Read the model definition and answer for the solid it produces. Units are mm, in the model's axes. Round coordinates to 2 decimals unless told otherwise and drop trailing zeros. Loops run counter-clockwise (first coordinate to the right, second up) from the corner with the lowest first, then second, coordinate; pieces in that order, holes last. Notation, with made-up numbers: (61.5, 60.5) - (115.5, 60.5) arc R21 ccw to (115.5, 78.5) - close; hole circle Ø2 at (25, -34). An arc over 180 degrees is marked (long way). Answer as CSV lines item,"result".
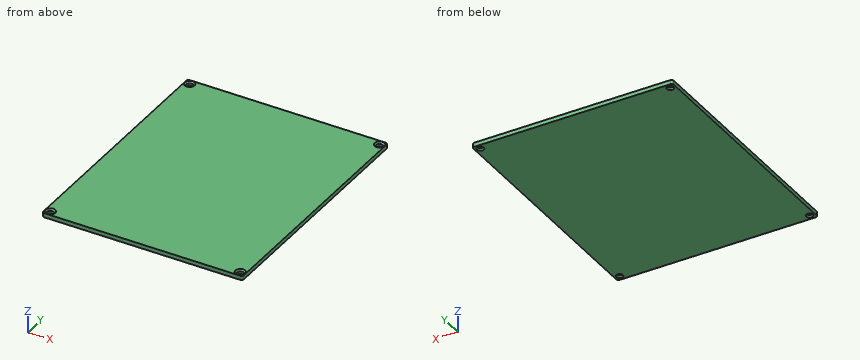
```python
from build123d import *

# Parameters (mm, degrees)
SKIZZE1_W                       = 96
SKIZZE1_H                       = 118
SKIZZE1_R                       = 1.6
AUFSATZ_LINEAR_AUSTRAGEN2_DEPTH = 2
FASE2_SIZE                      = 0.75
VERRUNDUNG2_R                   = 1


with BuildPart() as part:
    # Skizze1 → Aufsatz-Linear austragen2 (new body)
    with BuildSketch(Plane.XY):
        Rectangle(SKIZZE1_W, SKIZZE1_H)
        with Locations((-45.5, 56.5)):
            Circle(SKIZZE1_R, mode=Mode.SUBTRACT)
        with Locations((45.5, 56.5)):
            Circle(SKIZZE1_R, mode=Mode.SUBTRACT)
        with Locations((45.5, -56.5)):
            Circle(SKIZZE1_R, mode=Mode.SUBTRACT)
        with Locations((-45.5, -56.5)):
            Circle(SKIZZE1_R, mode=Mode.SUBTRACT)
    extrude(amount=AUFSATZ_LINEAR_AUSTRAGEN2_DEPTH)

    # Fase2
    fase2_edges = [part.edges().sort_by_distance(p)[0] for p in [
        (-47.1, 56.5, 2),
        (43.9, 56.5, 2),
        (43.9, -56.5, 2),
        (-47.1, -56.5, 2),
    ]]
    chamfer(fase2_edges, length=FASE2_SIZE)

    # Verrundung2
    verrundung2_edges = [part.edges().sort_by_distance(p)[0] for p in [
        (48, -59, 1),
        (-48, -59, 1),
        (-48, 59, 1),
        (48, 59, 1),
    ]]
    fillet(verrundung2_edges, radius=VERRUNDUNG2_R)


solid = part.part
```
1) Each of these flat-tipped pins is pushed along its axis until it touches: P1, Ø2.5, axis at x = -45.5, y = -56.5, coming from the +Z side (3 decimals); P2, Ø3.5, axis at x = -45.5, y = 56.5, coming from the +Z side. Where does it stop, or does it pass through?
Entries:
P1,"passes through"
P2,"stops at z = 1.4"
2) Find the intervals of material crossed by line 1 (Y direction, x = -45.5, z = 0.3), in increasing order.
Entries:
line 1,"y = -59 to -58.1, -54.9 to 54.9, 58.1 to 59"
3) A cutting plane is placed at A-A, the plane y = -56.5. Determine the outline of the cut face in (x, z).
Entries:
outline,"(-48, 0) - (-47.1, 0) - (-47.1, 1.25) - (-47.85, 2) - (-48, 2) - close; (-43.9, 0) - (43.9, 0) - (43.9, 1.25) - (43.15, 2) - (-43.15, 2) - (-43.9, 1.25) - close; (47.1, 0) - (48, 0) - (48, 2) - (47.85, 2) - (47.1, 1.25) - close"
4) A cutting plane is placed at B-B, the plane x = 45.5. Determine the outline of the cut face in (y, z).
Entries:
outline,"(-59, 0) - (-58.1, 0) - (-58.1, 1.25) - (-58.85, 2) - (-59, 2) - close; (-54.9, 0) - (54.9, 0) - (54.9, 1.25) - (54.15, 2) - (-54.15, 2) - (-54.9, 1.25) - close; (58.1, 0) - (59, 0) - (59, 2) - (58.85, 2) - (58.1, 1.25) - close"
